```python
from build123d import *

# Parameters (mm, degrees)
BOSS_EXTRUDE1_DEPTH                  = 7.62
SKETCH2_R                            = 18.415
BOSS_EXTRUDE2_DEPTH                  = 45.72
BOSS_EXTRUDE3_DEPTH                  = 15.24
SKETCH5_R                            = 6.35
BOSS_EXTRUDE4_DEPTH                  = 38.1
F_10_32_TAPPED_HOLE1_D               = 4.0386
F_10_32_TAPPED_HOLE1_DEPTH           = 7.62
F_10_32_TAPPED_HOLE1_TIP             = 1.213317848
F_10_32_TAPPED_HOLE1_ON_FACE_2_D     = 4.0386
F_10_32_TAPPED_HOLE1_ON_FACE_2_DEPTH = 7.62
F_10_32_TAPPED_HOLE1_ON_FACE_2_TIP   = 1.213317848
CUT_EXTRUDE1_START                   = -7.62
SKETCH8_R                            = 17.78
CUT_EXTRUDE1_DEPTH                   = 45.72
CUT_EXTRUDE2_REACH                   = 112.029
SKETCH9_R                            = 6
CUT_EXTRUDE3_DEPTH                   = 1.5875
F_10_32_TAPPED_HOLE2_D               = 4.0386
F_10_32_TAPPED_HOLE2_DEPTH           = 7.62
F_10_32_TAPPED_HOLE2_TIP             = 1.213317848
CUT_EXTRUDE4_DEPTH                   = 3.175
BOSS_EXTRUDE5_REACH                  = 61.758
SKETCH15_R                           = 1.5875
SKETCH16_R                           = 2.38125
BOSS_EXTRUDE6_DEPTH                  = 3.175


with BuildPart() as part:
    # Sketch1 → Boss-Extrude1 (new body)
    with BuildSketch(Plane(origin=(0, 0, 0), x_dir=(0, 0, -1), z_dir=(1, 0, 0))):
        with BuildLine():
            Line((-12.7, 19.05), (12.7, 19.05))
            ThreePointArc((12.7, 19.05), (17.190128061, 17.190128061), (19.05, 12.7))
            Line((19.05, 12.7), (19.05, -12.7))
            ThreePointArc((19.05, -12.7), (17.190128061, -17.190128061), (12.7, -19.05))
            Line((12.7, -19.05), (-12.7, -19.05))
            ThreePointArc((-12.7, -19.05), (-17.190128061, -17.190128061), (-19.05, -12.7))
            Line((-19.05, -12.7), (-19.05, 12.7))
            ThreePointArc((-19.05, 12.7), (-17.190128061, 17.190128061), (-12.7, 19.05))
        make_face()
    extrude(amount=BOSS_EXTRUDE1_DEPTH)

    # Sketch2 → Boss-Extrude2 (add)
    with BuildSketch(Plane(origin=(7.62, 0, 0), x_dir=(0, 0, -1), z_dir=(1, 0, 0))):
        with Locations(Location((0, 0, 0), (0, 0, 180))):
            Circle(SKETCH2_R)
    extrude(amount=BOSS_EXTRUDE2_DEPTH)

    # Sketch4 → Boss-Extrude3 (add)
    with BuildSketch(Plane(origin=(53.34, 0, 0), x_dir=(0, 0, -1), z_dir=(1, 0, 0))):
        with BuildLine():
            Line((12.7, 19.05), (-12.7, 19.05))
            ThreePointArc((-12.7, 19.05), (-17.190128061, 17.190128061), (-19.05, 12.7))
            Line((-19.05, 12.7), (-19.05, -12.7))
            ThreePointArc((-19.05, -12.7), (-17.190128061, -17.190128061), (-12.7, -19.05))
            Line((-12.7, -19.05), (12.7, -19.05))
            ThreePointArc((12.7, -19.05), (17.190128061, -17.190128061), (19.05, -12.7))
            Line((19.05, -12.7), (19.05, 12.7))
            ThreePointArc((19.05, 12.7), (17.190128061, 17.190128061), (12.7, 19.05))
        make_face()
    extrude(amount=BOSS_EXTRUDE3_DEPTH)

    # Sketch5 → Boss-Extrude4 (add)
    with BuildSketch(Plane(origin=(68.58, 0, 0), x_dir=(0, 0, -1), z_dir=(1, 0, 0))):
        with Locations(Location((0, 0, 0), (0, 0, 180))):
            Circle(SKETCH5_R)
    extrude(amount=BOSS_EXTRUDE4_DEPTH)

    # #10-32 Tapped Hole1
    with Locations(Plane(origin=(60.96, 9.525, -19.05), x_dir=(-1, 0, 0), z_dir=(0, 0, -1))):
        with Locations((0, 0), (0, -19.05), (57.15, 0), (57.15, -19.05)):
            Hole(F_10_32_TAPPED_HOLE1_D / 2, depth=F_10_32_TAPPED_HOLE1_DEPTH)
            with Locations((0, 0, -(F_10_32_TAPPED_HOLE1_DEPTH + F_10_32_TAPPED_HOLE1_TIP / 2))):  # 118° drill point
                Cone(0, F_10_32_TAPPED_HOLE1_D / 2, F_10_32_TAPPED_HOLE1_TIP, mode=Mode.SUBTRACT)

    # #10-32 Tapped Hole1 on face 2
    with Locations(Plane(origin=(60.96, 9.525, 19.05), x_dir=(1, 0, 0), z_dir=(0, 0, 1))):
        with Locations((0, 0), (0, -19.05), (-57.15, 0), (-57.15, -19.05)):
            Hole(F_10_32_TAPPED_HOLE1_ON_FACE_2_D / 2, depth=F_10_32_TAPPED_HOLE1_ON_FACE_2_DEPTH)
            with Locations((0, 0, -(F_10_32_TAPPED_HOLE1_ON_FACE_2_DEPTH + F_10_32_TAPPED_HOLE1_ON_FACE_2_TIP / 2))):  # 118° drill point
                Cone(0, F_10_32_TAPPED_HOLE1_ON_FACE_2_D / 2, F_10_32_TAPPED_HOLE1_ON_FACE_2_TIP, mode=Mode.SUBTRACT)

    # Sketch8 → Cut-Extrude1 (cut)
    with BuildSketch(Plane.ZY.offset(CUT_EXTRUDE1_START)):
        Circle(SKETCH8_R)
    extrude(amount=-CUT_EXTRUDE1_DEPTH, mode=Mode.SUBTRACT)

    # Sketch9 → Cut-Extrude2 (cut, up to next)
    with BuildSketch(Plane.ZY, mode=Mode.PRIVATE) as cut_extrude2_sk1:
        Circle(SKETCH9_R)
    cut_extrude2_tool1 = extrude(cut_extrude2_sk1.sketch, amount=-CUT_EXTRUDE2_REACH, mode=Mode.PRIVATE) & part.part
    add(cut_extrude2_tool1.solids().sort_by_distance((0, 0, 0))[0], mode=Mode.SUBTRACT)

    # Sketch10 → Cut-Extrude3 (cut, symmetric)
    with BuildSketch(Plane.XY):
        Polygon((106.68, 4.7625), (81.28, 4.7625), (78.105, 6.35), (106.68, 6.35), align=None)
    extrude(amount=CUT_EXTRUDE3_DEPTH, both=True, mode=Mode.SUBTRACT)

    # #10-32 Tapped Hole2
    with Locations(Plane(origin=(106.68, 0, 0), x_dir=(0, 0, -1), z_dir=(1, 0, 0))):
        with Locations((0, 0)):
            Hole(F_10_32_TAPPED_HOLE2_D / 2, depth=F_10_32_TAPPED_HOLE2_DEPTH)
            with Locations((0, 0, -(F_10_32_TAPPED_HOLE2_DEPTH + F_10_32_TAPPED_HOLE2_TIP / 2))):  # 118° drill point
                Cone(0, F_10_32_TAPPED_HOLE2_D / 2, F_10_32_TAPPED_HOLE2_TIP, mode=Mode.SUBTRACT)

    # Sketch14 → Cut-Extrude4 (cut)
    with BuildSketch(Plane(origin=(68.58, 0, 0), x_dir=(0, 0, -1), z_dir=(1, 0, 0))):
        with BuildLine():
            Line((-14.2875, 11.1125), (-19.05, 11.1125))
            Line((-19.05, 11.1125), (-19.05, 19.05))
            Line((-19.05, 19.05), (-11.1125, 19.05))
            Line((-11.1125, 19.05), (-11.1125, 14.2875))
            ThreePointArc((-11.1125, 14.2875), (-12.04243597, 12.04243597), (-14.2875, 11.1125))
        make_face()
        with BuildLine():
            Line((-14.2875, -11.1125), (-19.05, -11.1125))
            Line((-19.05, -11.1125), (-19.05, -19.05))
            Line((-19.05, -19.05), (-11.1125, -19.05))
            Line((-11.1125, -19.05), (-11.1125, -14.2875))
            ThreePointArc((-11.1125, -14.2875), (-12.04243597, -12.04243597), (-14.2875, -11.1125))
        make_face()
        with BuildLine():
            Line((11.1125, 14.2875), (11.1125, 19.05))
            Line((11.1125, 19.05), (19.05, 19.05))
            Line((19.05, 19.05), (19.05, 11.1125))
            Line((19.05, 11.1125), (14.2875, 11.1125))
            ThreePointArc((14.2875, 11.1125), (12.04243597, 12.04243597), (11.1125, 14.2875))
        make_face()
        with BuildLine():
            Line((14.2875, -11.1125), (19.05, -11.1125))
            Line((19.05, -11.1125), (19.05, -19.05))
            Line((19.05, -19.05), (11.1125, -19.05))
            Line((11.1125, -19.05), (11.1125, -14.2875))
            ThreePointArc((11.1125, -14.2875), (12.04243597, -12.04243597), (14.2875, -11.1125))
        make_face()
    extrude(amount=-CUT_EXTRUDE4_DEPTH, mode=Mode.SUBTRACT)

    # Sketch15 → Boss-Extrude5 (add, up to next)
    with BuildSketch(Plane.ZY.offset(-53.34), mode=Mode.PRIVATE) as boss_extrude5_sk1:
        with Locations(Location((14.2875, 14.2875, 0), (0, 0, 180))):
            Circle(SKETCH15_R)
    boss_extrude5_tool1 = extrude(boss_extrude5_sk1.sketch, amount=BOSS_EXTRUDE5_REACH, mode=Mode.PRIVATE) - part.part
    # Sketch15 → Boss-Extrude5 (add, up to next)
    with BuildSketch(Plane.ZY.offset(-53.34), mode=Mode.PRIVATE) as boss_extrude5_sk2:
        with Locations(Location((-14.2875, 14.2875, 0), (0, 0, 180))):
            Circle(SKETCH15_R)
    boss_extrude5_tool2 = extrude(boss_extrude5_sk2.sketch, amount=BOSS_EXTRUDE5_REACH, mode=Mode.PRIVATE) - part.part
    # Sketch15 → Boss-Extrude5 (add, up to next)
    with BuildSketch(Plane.ZY.offset(-53.34), mode=Mode.PRIVATE) as boss_extrude5_sk3:
        with Locations(Location((14.2875, -14.2875, 0), (0, 0, 180))):
            Circle(SKETCH15_R)
    boss_extrude5_tool3 = extrude(boss_extrude5_sk3.sketch, amount=BOSS_EXTRUDE5_REACH, mode=Mode.PRIVATE) - part.part
    # Sketch15 → Boss-Extrude5 (add, up to next)
    with BuildSketch(Plane.ZY.offset(-53.34), mode=Mode.PRIVATE) as boss_extrude5_sk4:
        with Locations(Location((-14.2875, -14.2875, 0), (0, 0, 180))):
            Circle(SKETCH15_R)
    boss_extrude5_tool4 = extrude(boss_extrude5_sk4.sketch, amount=BOSS_EXTRUDE5_REACH, mode=Mode.PRIVATE) - part.part
    add(boss_extrude5_tool1.solids().sort_by_distance((53.34, 14.2875, 14.2875))[0])
    add(boss_extrude5_tool2.solids().sort_by_distance((53.34, 14.2875, -14.2875))[0])
    add(boss_extrude5_tool3.solids().sort_by_distance((53.34, -14.2875, 14.2875))[0])
    add(boss_extrude5_tool4.solids().sort_by_distance((53.34, -14.2875, -14.2875))[0])

    # Sketch16 → Boss-Extrude6 (add)
    with BuildSketch(Plane(origin=(65.405, 0, 0), x_dir=(0, 0, -1), z_dir=(1, 0, 0))):
        with Locations((-14.2875, 14.2875)):
            Circle(SKETCH16_R)
        with Locations((-14.2875, -14.2875)):
            Circle(SKETCH16_R)
        with Locations((14.2875, -14.2875)):
            Circle(SKETCH16_R)
        with Locations((14.2875, 14.2875)):
            Circle(SKETCH16_R)
    extrude(amount=BOSS_EXTRUDE6_DEPTH)


solid = part.part
```
Work out the finished part from the listing and answer in its coordinate system (mm). A direction names the side the tool comes from. Coordinates: 2 decimals unless noted, no trailing zeros. Write each loop counter-clockwise with the first axis right and the second up, starting at its lowest first coordinate (ties: lowest second). Pieces come first, ordered by that corner, then holes.
Q1. A cutting plane is placed at A-A, the plane x = 49. Give the vertices of the cut face in (y, z) (1 decimal).
Q2. Each of these flat-tipped pins is pushed along its axis until it touches: pin 1 Ø10 at (x, y) = (37.5, -1) entering from +Z (3 decimals); pin 2 Ø3 at (y, z) = (0, 0) entering from -X; pin 3 Ø5 at (x, y) = (16.5, -15) entering from -Z (3 decimals). Where does it stop, or does it pass through?
Q3. A cutting plane is placed at C-C, the plane x = 87. Give the vertices of the cut face in (y, z).
Q4. Find the intervals of material crossed by line 1 (X direction, y = -12, z = 0); line 2 (Y direction, x = 60.96, z = -14.75); line 3 (X direction, y = 10, z = 15.5), in increasing order.
Q5. Determine the mould class of faces 1 (the face through (1.945, 8.752, 15.187)), 2 (the face through (59.29, 17.14, -17.24)), 3 (the face through (68.58, -14, 14)) for opening direction X: released by +X, released by -X, zero draft, split by the parting line, or undercut.
Q6. A cutting plane is placed at B-B, the plane y = -4. Give the vertices of the cut face in (x, z).
Q7. Which of the six approach directions +Z, -Z, +X, -X, +Y, -Y give full straight-line access (tool end or side, diameter ignored) to faces 4 (the face through (30.8, 14.22, -12.7)), 5 (the face through (59.095, -10.298, 15.187)), 6 (the face through (62.825, -10.298, -15.187)), 7 (the face through (67, 17, -11.112))?
Findings below:
1. outline: circle Ø36.8 at (0, 0); circle Ø3.2 at (-14.3, -14.3); circle Ø3.2 at (-14.3, 14.3); circle Ø3.2 at (14.3, -14.3); circle Ø3.2 at (14.3, 14.3); hole circle Ø35.6 at (0, 0)
2. pin 1: stops at z = 18.415
2. pin 2: stops at x = 53.34
2. pin 3: stops at z = -15.875
3. outline: (4.76, -1.59) - (4.76, 1.59) - (6.15, 1.59) arc R6.35 ccw (long way) to (6.15, -1.59) - close
4. line 1: x = 0 to 7.62, 53.34 to 68.58
4. line 2: y = -18.71 to -11.54, -7.51 to 7.51, 11.54 to 18.71
4. line 3: x = 0 to 1.85, 5.77 to 7.62, 53.34 to 59, 62.92 to 68.58
5. face 1: undercut
5. face 2: zero draft
5. face 3: released by +X
6. outline: (0, -19.05) - (7.62, -19.05) - (7.62, -17.98) - (53.34, -17.98) - (53.34, -19.05) - (68.58, -19.05) - (68.58, -4.93) - (106.68, -4.93) - (106.68, 4.93) - (68.58, 4.93) - (68.58, 19.05) - (53.34, 19.05) - (53.34, 17.98) - (7.62, 17.98) - (7.62, 19.05) - (0, 19.05) - (0, 4.47) - (7.62, 4.47) - (7.62, 17.32) - (53.34, 17.32) - (53.34, -17.32) - (7.62, -17.32) - (7.62, -4.47) - (0, -4.47) - close
7. face 4: none
7. face 5: +Z
7. face 6: -Z
7. face 7: +X, +Y
